Study the drawing (mm; zero at the part's minimum x, y, z) and answer. Coordinates: 2 decimals unless noted, no trailing zeros. Loops run counter-clockwise (first coordinate to the right, second up) from the corner with the lowest first, then second, coordinate; pieces in that order, holes last. Notation, with made-up numbers: (51.25, 69) -> (98.25, 69) arc R28 cw to (98.25, 93) -> close; hole circle Ø6 at (-32.75, 15). An arc over 180 degrees is marked (long way). Answer as a JSON object with one key per item and string values. Group by question number.
Q1. The part is cut by section C-C on x = 23. Write down the section's boundary in (y, z), and give its area (3 significant figures).
Q2. A straight line is drawn through the part: line 1 along Y through (x, z) = (25, 1). Find the intervals that lie inside material, in ascending order. Write a range as [from, to].
Q3. The part is cut by section B-B on x = 105. Write down the section's boundary in (y, z), and give its area (3 significant figures).
Q4. The part is cut by section A-A on y = 45. Write down the section's boundary in (x, z).
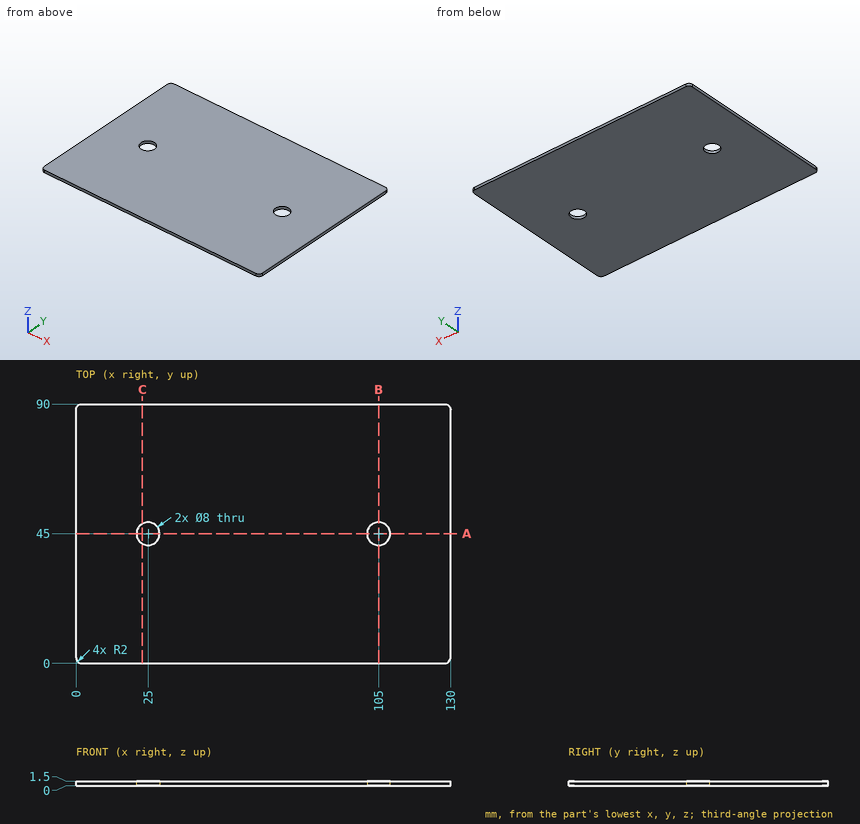
Final values:
{
 "1": {"outline": "(0, 0) -> (41.54, 0) -> (41.54, 1.5) -> (0, 1.5) -> close; (48.46, 0) -> (90, 0) -> (90, 1.5) -> (48.46, 1.5) -> close", "area": "125 mm2"},
 "2": {"line 1": "y = [0, 41], [49, 90]"},
 "3": {"outline": "(0, 0) -> (41, 0) -> (41, 1.5) -> (0, 1.5) -> close; (49, 0) -> (90, 0) -> (90, 1.5) -> (49, 1.5) -> close", "area": "123 mm2"},
 "4": {"outline": "(0, 0) -> (21, 0) -> (21, 1.5) -> (0, 1.5) -> close; (29, 0) -> (101, 0) -> (101, 1.5) -> (29, 1.5) -> close; (109, 0) -> (130, 0) -> (130, 1.5) -> (109, 1.5) -> close"}
}
